```python
from build123d import *

# Parameters (mm, degrees)
SKETCH1_R           = 1.778
SKETCH1_W           = 9.525
SKETCH1_H           = 3.175
BOSS_EXTRUDE1_DEPTH = 3.175


with BuildPart() as part:
    # Sketch1 → Boss-Extrude1 (new body)
    with BuildSketch(Plane(origin=(0, 0, 0), x_dir=(1, 0, 0), z_dir=(0, 1, 0))):
        Polygon((0, 0), (0, 12.7), (-5.08, 12.7), (-5.08, 25.4), (0, 25.4), (0, 38.1), (38.1, 38.1), (38.1, 25.4), (43.18, 25.4), (43.18, 12.7), (38.1, 12.7), (38.1, 0), align=None)
        with Locations(Location((-2.54, 19.05, 0), (0, 0, 270))):
            Circle(SKETCH1_R, mode=Mode.SUBTRACT)
        with Locations(Location((40.64, 19.05, 0), (0, 0, 270))):
            Circle(SKETCH1_R, mode=Mode.SUBTRACT)
        with Locations((14.2875, 4.7625)):
            Rectangle(SKETCH1_W, SKETCH1_H, mode=Mode.SUBTRACT)
    extrude(amount=BOSS_EXTRUDE1_DEPTH)


solid = part.part
```
Can you work these out from the model? Positions are in its coordinate system, mm. A direction names the side the tool comes from. Coordinates: 2 decimals unless noted, no trailing zeros. Loops run counter-clockwise (first coordinate to the right, second up) from the corner with the lowest first, then second, coordinate; pieces in that order, holes last. Notation, with made-up numbers: (17.25, 11) - (58.25, 11) arc R24 ccw to (58.25, 45) - close; hole circle Ø1 at (76.25, 24). An arc over 180 degrees is marked (long way). Answer as CSV lines item,"result". Start each with the question number.
1) Suppose I cut it at B-B (z = -4). Please give me the cut outline in (x, y) (3 decimals), plus the area to 3 significant figures.
2) Which directions (+Z, -Z, +X, -X, +Y, -Y) give clear straight access to the entire face, cutting with the end or side of a thin tool? Please do faces 4 (the flat face through (38.1, 2, -32)), 5 (the flat face through (19.05, 2, -5)), 6 (the flat face through (41, 2, -12.7)), 7 (the flat face through (-3, 2, -12.7)), 8 (the flat face through (0, 2, -32)).
3) Suppose I cut it at D-D (z = -19.05). Please give me the cut outline in (x, y) (3 decimals).
4) I need wall thicknesses on line 1 (X direction, y = 2.5, z = -19.05); line 2 (X direction, y = 1.85, z = -5.5) (3 decimals); line 3 (Z direction, x = 12, y = 1.15) (3 decimals). Which ranges of each line are inside material? Lowest first, please. Write a range as from..to.
5) Suppose I cut it at C-C (y = 1.5). Please give me the cut outline in (x, z) (3 decimals), plus the area to 3 significant figures.
6) Thinking about a two-plate mould opening in Z: for faces 1 (the flat face through (43.18, 2, -19)), 2 (the flat face through (41, 2, -25.4)), 3 (the cylindrical face through (39.56, 1.57, -20.46)), which applies, pulls with the +Z half, pulls with the -Z half, needs draft (parallel to the pull), parting line crosses it, or undercut?
7) Suppose I cut it at A-A (x = 40.64). Please give me the cut outline in (y, z) (3 decimals).
8) For pin 1 (1.6 mm diameter, centred on x = 40, y = 2, fed in from -Z); pin 2 (1.6 mm diameter, centred on y = 1.5, z = -5.5, fed in from -X), each with a flat end and sliding along its axis, tell me the tip position at first contact or that it passes through.
Check result:
1,outline,"(0, 0) - (9.525, 0) - (9.525, 3.175) - (0, 3.175) - close; (19.05, 0) - (38.1, 0) - (38.1, 3.175) - (19.05, 3.175) - close"
1,area,"90.7 mm²"
2,face 4,"-Z, +X, +Y, -Y"
2,face 5,"+Y, -Y"
2,face 6,"+Z, +X, +Y, -Y"
2,face 7,"+Z, -X, +Y, -Y"
2,face 8,"-Z, -X, +Y, -Y"
3,outline,"(-5.08, 0) - (-4.318, 0) - (-4.318, 3.175) - (-5.08, 3.175) - close; (-0.762, 0) - (38.862, 0) - (38.862, 3.175) - (-0.762, 3.175) - close; (42.418, 0) - (43.18, 0) - (43.18, 3.175) - (42.418, 3.175) - close"
4,line 1,"x = -5.08..-4.32, -0.76..38.86, 42.42..43.18"
4,line 2,"x = 0..9.525, 19.05..38.1"
4,line 3,"z = -38.1..-6.35, -3.175..0"
5,outline,"(-5.08, -25.4) - (0, -25.4) - (0, -38.1) - (38.1, -38.1) - (38.1, -25.4) - (43.18, -25.4) - (43.18, -12.7) - (38.1, -12.7) - (38.1, 0) - (0, 0) - (0, -12.7) - (-5.08, -12.7) - close; hole circle Ø3.556 at (-2.54, -19.05); hole (9.525, -6.35) - (19.05, -6.35) - (19.05, -3.175) - (9.525, -3.175) - close; hole circle Ø3.556 at (40.64, -19.05)"
5,area,"1,530 mm²"
6,face 1,"needs draft"
6,face 2,"pulls with the -Z half"
6,face 3,"undercut"
7,outline,"(0, -25.4) - (3.175, -25.4) - (3.175, -20.828) - (0, -20.828) - close; (0, -17.272) - (3.175, -17.272) - (3.175, -12.7) - (0, -12.7) - close"
8,pin 1,"stops at z = -25.4"
8,pin 2,"stops at x = 0"
